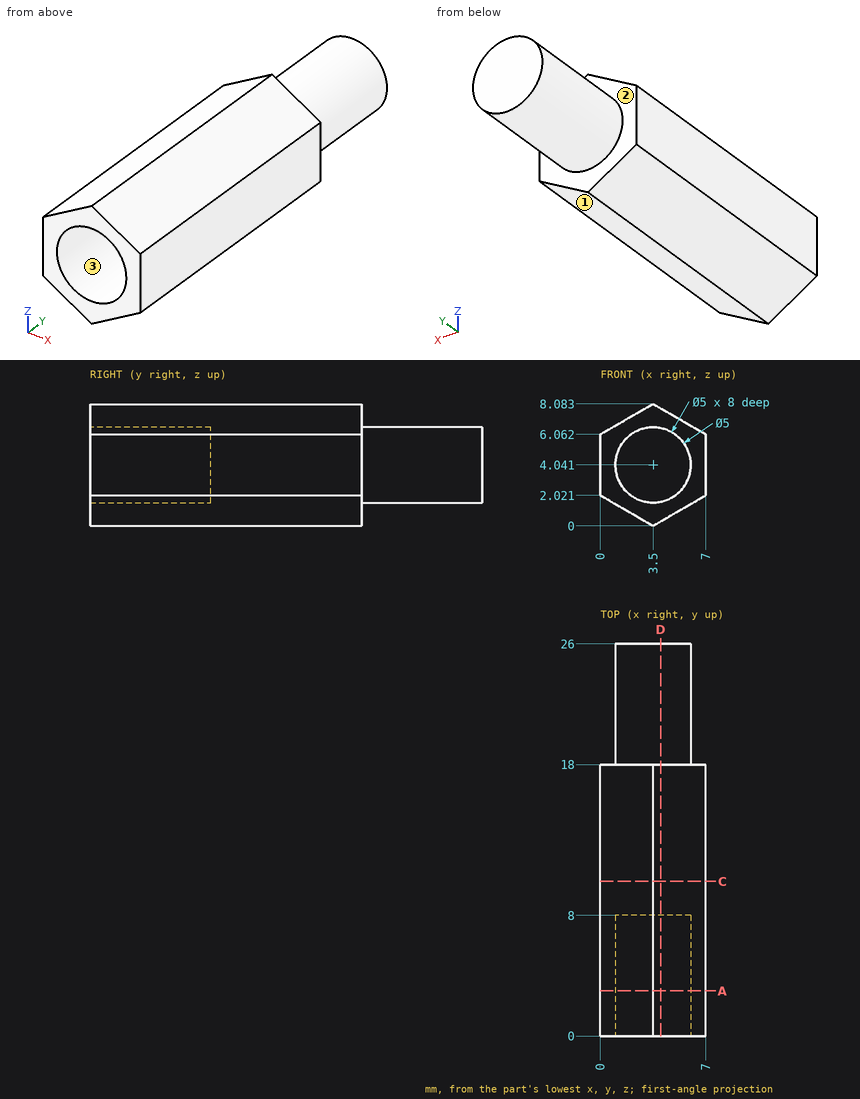
Source: three-view drawing plus pictorial views. Frame: mm from the lowest corner of the part. A direction names the side the tool comes from. Round coordinates to 2 decimals unless told otherwise and drop trailing zeros. Order: outer loops, then holes, each group sorted by start corner. A loop starts at its lowest first (then second) coordinate and runs counter-clockwise, first axis right, second up. Notation, with made-up numbers: M 2.5,69.5 L 51.5,69.5 A33 cw 51.5,108.5 Z; hole C -29,17.5 d11. An arc over 180 degrees is marked long. One line per item, written item: value.
(1) Line query: probe 1 along Y at (x, z) = (2.5, 5); probe 2 along X at (y, z) = (4.5, 3); probe 3 along X at (y, z) = (5.75, 4.25). Output: solid intervals per line, ascending. Write a range as [from, to].
Result sheet:
probe 1: [8, 26]
probe 2: [0, 1.23], [5.77, 7]
probe 3: [0, 1.01], [5.99, 7]
(2) Cut plane D-D (x = 4). Return the cut outline in (y, z) (1 decimal).
Result sheet:
outline: M 0,0.3 L 18,0.3 L 18,1.6 L 26,1.6 L 26,6.5 L 18,6.5 L 18,7.8 L 0,7.8 L 0,6.5 L 8,6.5 L 8,1.6 L 0,1.6 Z
(3) Reachability of the marked faces 1, 2 and 3 from +Z, -Z, +X, -X, +Y, -Y: full face, straight path, thin tool, end or side. Return the list, or none.
Result sheet:
face 1: -Z, +X, +Y, -Y
face 2: +Y
face 3: -Y
(4) Cut plane A-A (y = 3). Return the cut outline in (x, z), and give its area (3 significant figures).
Result sheet:
outline: M 0,2.02 L 3.5,0 L 7,2.02 L 7,6.06 L 3.5,8.08 L 0,6.06 Z; hole C 3.5,4.04 d5
area: 22.8 mm2
(5) Cut plane C-C (y = 10.25). Return the cut outline in (x, z).
Result sheet:
outline: M 0,2.02 L 3.5,0 L 7,2.02 L 7,6.06 L 3.5,8.08 L 0,6.06 Z
(6) Pin query (flat end, axial travel): P1, Ø2.5, axis at x = 3.5, z = 5, coming from the -Y side; P2, Ø3, axis at x = 2, y = 21.5, coming from the +Z side; P3, Ø1.5, axis at x = 2, y = 17, coming from the +Z side. Return the tip coordinate at first contact, or that it passes through.
Result sheet:
P1: y = 8
P2: z = 6.54
P3: z = 7.65
